Build history of the part. All positions in model axes, mm. A direction names the side the tool comes from. Give positions to 0.01 mm unless a question says otherwise; leave off trailing zeros. Write each loop counter-clockwise with the first axis right and the second up, starting at its lowest first coordinate (ties: lowest second). Pieces come first, ordered by that corner, then holes. Notation, with made-up numbers: M 46,-27 L 59,-27 A31 cw 59,4 Z; hole C 72.5,41 d6. An arc over 180 degrees is marked long. One line per item, written item: value. Start each with the question number.
Autodesk Inventor part; units mm, degrees
ref_plane "YZ Plane" through (0, 0, 0) normal (1, 0, 0) x (0, 1, 0)
ref_plane "XZ Plane" through (0, 0, 0) normal (0, 1, 0) x (-1, 0, 0)
ref_plane "XY Plane" through (0, 0, 0) normal (0, 0, 1) x (1, 0, 0)
sketch "Sketch1" plane through (0, 0, 0) normal (0, 1, 0) x (-1, 0, 0)
  line L0 (0, 0) -> (-42, 0)
  line L1 (-42, 0) -> (-42, -80)
  line L2 (-42, -80) -> (0, -80)
  line L3 (0, 0) -> (0, -5)
  line L4 (0, -5) -> (3, -5)
  line L5 (3, -5) -> (3, -25)
  line L6 (3, -25) -> (0, -25)
  line L7 (0, -80) -> (0, -75)
  line L8 (0, -75) -> (3, -75)
  line L9 (3, -75) -> (3, -55)
  line L10 (3, -55) -> (0, -55)
  line L11 (0, -25) -> (0, -30)
  line L12 (0, -30) -> (3, -30)
  line L13 (3, -30) -> (3, -50)
  line L14 (3, -50) -> (0, -50)
  line L15 (0, -50) -> (0, -55)
  line L16 (0, -40) -> (0, -13) construction
  line L17 (0, -13) -> (-32.5, -13) construction
  line L18 (-32.5, -13) -> (-36.5, -13) construction
  line L19 (-36.5, -13) -> (-36.5, -9) construction
  line L20 (-36.5, -9) -> (-32.5, -9) construction
  line L21 (-32.5, -9) -> (-32.5, -13) construction
  circle A0 centre (-34.5, -11) radius 2
  line L22 (-32.5, -13) -> (-32.5, -67) construction
  line L23 (-32.5, -67) -> (-37, -67) construction
  line L24 (-37, -67) -> (-37, -71.5) construction
  line L25 (-37, -71.5) -> (-32.5, -71.5) construction
  line L26 (-32.5, -71.5) -> (-32.5, -67) construction
  circle A1 centre (-34.75, -69.25) radius 2.25
  point P0 (-36.5, -11)
  point P1 (-37, -69.25)
  dimension "d1" = 80
  dimension "d2" = 5
  dimension "d3" = 3
  dimension "d4" = 20
  dimension "d5" = 5
  dimension "d6" = 20
  dimension "d7" = 5
  dimension "d8" = 20
  dimension "d12" = 27
  dimension "d13" = 32.5
  dimension "d14" = 4
  dimension "d15" = 4
  dimension "d16" = 54
  dimension "d17" = 4.5
  dimension "d18" = 4.5
  dimension "d20" = 5
  dimension "d21" = 0
  dimension "d22" = 3
  dimension "d23" = 0
extrude "Extrusion1" add sketch "Sketch1" along normal blind 3
1) Band-saw the part on A-A (z = -11). List the corners of the cut face in (x, y), then the cut area to 3 significant figures.
2) Tool access for faces 1 (the face through (-1, 1, -75)), 2 (the face through (-1, 1, -5)), 3 (the face through (21, 1, -80)), 4 (the face through (-2, 1, -50)), 5 (the face through (20, 3, -39)): list every direction of +Z, -Z, +X, -X, +Y, -Y with a clear straight run to the whole face (end or side of a thin tool).
3) Drop flat-ended pins along their axis: P1, Ø3, axis at x = 31, z = -13, coming from the -Y side; P2, Ø1.5, axis at y = 1.5, z = -2.5, coming from the -X side; P3, Ø3.5, axis at x = 34.5, z = -11, coming from the -Y side; P4, Ø0.9, axis at x = -1, y = 1.5, coming from the +Z side. Give the stop position or say it passes through.
4) Band-saw the part on D-D (z = -69.25). List the corners of the cut face in (x, y).
5) Mould opens along X. For faces 6 (the face through (-3, 1, -40)), 7 (the face through (21, 1, 0)), 8 (the face through (32.592, 1.479, -11.601)) say: released by +X, released by -X, zero draft, split by the parting line, or undercut.
6) Band-saw the part on C-C (x = 34.5). List the corners of the cut face in (y, z).
7) Probe line 1 along Z through (x, y) = (-1, 1.45); line 2 along Z through (x, y) = (34.75, 1); line 3 along X through (y, z) = (0.5, -4). List the from-to ranges inside material, lowest first. Write a range as from..to.
8) Band-saw the part on B-B (y = 1.35). List the corners of the cut face in (x, z).
Model answer:
1. outline: M -3,0 L 32.5,0 L 32.5,3 L -3,3 Z; M 36.5,0 L 42,0 L 42,3 L 36.5,3 Z
1. area: 123 mm²
2. face 1: -Z, -X, +Y, -Y
2. face 2: +Z, -X, +Y, -Y
2. face 3: -Z, +X, -X, +Y, -Y
2. face 4: -X, +Y, -Y
2. face 5: +Z, -Z, +X, -X, +Y
3. P1: stops at y = 0
3. P2: stops at x = 0
3. P3: passes through
3. P4: stops at z = -5
4. outline: M -3,0 L 32.5,0 L 32.5,3 L -3,3 Z; M 37,0 L 42,0 L 42,3 L 37,3 Z
5. face 6: released by -X
5. face 7: zero draft
5. face 8: undercut
6. outline: M 0,-80 L 3,-80 L 3,-71.49 L 0,-71.49 Z; M 0,-67.01 L 3,-67.01 L 3,-13 L 0,-13 Z; M 0,-9 L 3,-9 L 3,0 L 0,0 Z
7. line 1: z = -75..-55, -50..-30, -25..-5
7. line 2: z = -80..-71.5, -67..-12.98, -9.02..0
7. line 3: x = 0..42
8. outline: M -3,-75 L 0,-75 L 0,-80 L 42,-80 L 42,0 L 0,0 L 0,-5 L -3,-5 L -3,-25 L 0,-25 L 0,-30 L -3,-30 L -3,-50 L 0,-50 L 0,-55 L -3,-55 Z; hole C 34.75,-69.25 d4.5; hole C 34.5,-11 d4
